```python
from build123d import *

# Parameters (mm, degrees)
SKETCH1_W           = 86.36
SKETCH1_H           = 76.2
SKETCH1_R           = 2.2225
SKETCH1_W_2         = 8.255
SKETCH1_R_2         = 1.016
BOSS_EXTRUDE1_DEPTH = 3.175
SKETCH2_W           = 102.87
SKETCH2_H           = 76.2
SKETCH2_W_2         = 100.33
SKETCH2_H_2         = 72.39
BOSS_EXTRUDE3_DEPTH = 12.7


with BuildPart() as part:
    # Sketch1 → Boss-Extrude1 (new body)
    # profile 1 of 3: a face of its own
    with BuildSketch(Plane(origin=(0, 0, 0), x_dir=(1, 0, 0), z_dir=(0, 1, 0))):
        Rectangle(SKETCH1_W, SKETCH1_H)
        with Locations(Location((-38.1, -10.16, 0), (0, 0, 270))):
            Circle(SKETCH1_R, mode=Mode.SUBTRACT)
        with Locations(Location((-38.1, 10.16, 0), (0, 0, 270))):
            Circle(SKETCH1_R, mode=Mode.SUBTRACT)
        with Locations(Location((38.1, -10.16, 0), (0, 0, 270))):
            Circle(SKETCH1_R, mode=Mode.SUBTRACT)
        with Locations(Location((38.1, 10.16, 0), (0, 0, 270))):
            Circle(SKETCH1_R, mode=Mode.SUBTRACT)
    # profile 2 of 3: a face of its own
    with BuildSketch(Plane(origin=(0, 0, 0), x_dir=(1, 0, 0), z_dir=(0, 1, 0))):
        with Locations((-47.3075, 0)):
            Rectangle(SKETCH1_W_2, SKETCH1_H)
        with Locations(Location((-46.355, 31.369, 0), (0, 0, 270))):
            Circle(SKETCH1_R_2, mode=Mode.SUBTRACT)
        with Locations(Location((-46.355, -31.369, 0), (0, 0, 270))):
            Circle(SKETCH1_R_2, mode=Mode.SUBTRACT)
    # profile 3 of 3: a face of its own
    with BuildSketch(Plane(origin=(0, 0, 0), x_dir=(1, 0, 0), z_dir=(0, 1, 0))):
        with Locations((47.3075, 0)):
            Rectangle(SKETCH1_W_2, SKETCH1_H)
        with Locations(Location((46.355, -31.369, 0), (0, 0, 270))):
            Circle(SKETCH1_R_2, mode=Mode.SUBTRACT)
        with Locations(Location((46.355, 31.369, 0), (0, 0, 270))):
            Circle(SKETCH1_R_2, mode=Mode.SUBTRACT)
    extrude(amount=BOSS_EXTRUDE1_DEPTH)

    # Sketch2 → Boss-Extrude3 (add)
    with BuildSketch(Plane(origin=(0, 3.175, 0), x_dir=(1, 0, 0), z_dir=(0, 1, 0))):
        Rectangle(SKETCH2_W, SKETCH2_H)
        Rectangle(SKETCH2_W_2, SKETCH2_H_2, mode=Mode.SUBTRACT)
    extrude(amount=BOSS_EXTRUDE3_DEPTH)


solid = part.part
```
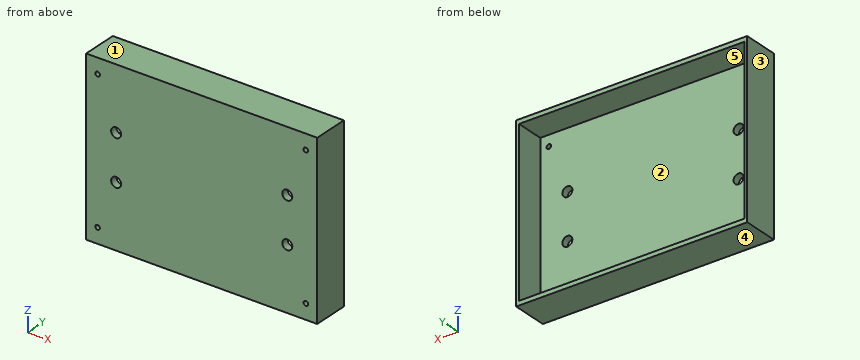
For this review, take the finished solid that the model builds, in its own axes (mm). Face numbers are marked on the shaded views. A direction names the side the tool comes from. Round coordinates to 2 decimals unless told otherwise and drop trailing zeros. Write each loop counter-clockwise with the first axis right and the second up, starting at its lowest first coordinate (ties: lowest second). Pieces come first, ordered by that corner, then holes. Notation, with made-up numbers: (-35, 12.25) - (-14, 12.25) arc R6 cw to (-14, 18.25) - close; hole circle Ø5 at (6, 35). An arc over 180 degrees is marked (long way). Put each result on its own line as item: value.
Q1. Machinability: for the marked faces 4 and 5, which of the approach directions +Z, -Z, +X, -X, +Y, -Y give a long, thin tool a straight path to every point of the face, cutting with its end or side? Answer none if there is none.
Solved:
face 4: -Z, +X, -X, +Y, -Y
face 5: +Y
Q2. We need section A-A (x = -38.1). Give the boundary of the cut face in (y, z) (1 decimal), and give its area (3 significant figures).
Solved:
outline: (0, -38.1) - (15.9, -38.1) - (15.9, -36.2) - (3.2, -36.2) - (3.2, -12.4) - (0, -12.4) - close; (0, -7.9) - (3.2, -7.9) - (3.2, 7.9) - (0, 7.9) - close; (0, 12.4) - (3.2, 12.4) - (3.2, 36.2) - (15.9, 36.2) - (15.9, 38.1) - (0, 38.1) - close
area: 262 mm2
Q3. Insertion check: pin 1 Ø6 at (x, z) = (38.1, 10.16) entering from +Y (3 decimals). The pin has a flat end and moves straight along its axis. Give the tip position at first contact, or say it passes through.
Solved:
pin 1: stops at y = 3.175
Q4. Wall thickness on probe 1 along X at (y, z) = (1.1, 10.16) (1 decimal); probe 2 along Z at (x, y) = (41.5, 11) (3 decimals); probe 3 along X at (y, z) = (4.25, -6) (3 decimals): over which ranges is each line inside the solid? List them lowest first.
Solved:
probe 1: x = -51.4 to -40.3, -35.9 to 35.9, 40.3 to 51.4
probe 2: z = -38.1 to -36.195, 36.195 to 38.1
probe 3: x = -51.435 to -50.165, 50.165 to 51.435
Q5. We need section D-D (x = 0). Give the boundary of the cut face in (y, z) (3 decimals).
Solved:
outline: (0, -38.1) - (15.875, -38.1) - (15.875, -36.195) - (3.175, -36.195) - (3.175, 36.195) - (15.875, 36.195) - (15.875, 38.1) - (0, 38.1) - close
Q6. We need section B-B (z = -10.16). Give the boundary of the cut face in (x, y) (1 decimal), and give its area (3 significant figures).
Solved:
outline: (-51.4, 0) - (-40.3, 0) - (-40.3, 3.2) - (-50.2, 3.2) - (-50.2, 15.9) - (-51.4, 15.9) - close; (-35.9, 0) - (35.9, 0) - (35.9, 3.2) - (-35.9, 3.2) - close; (40.3, 0) - (51.4, 0) - (51.4, 15.9) - (50.2, 15.9) - (50.2, 3.2) - (40.3, 3.2) - close
area: 331 mm2
Q7. We need section C-C (y = 9). Give the boundary of the cut face in (x, z) (3 decimals).
Solved:
outline: (-51.435, -38.1) - (51.435, -38.1) - (51.435, 38.1) - (-51.435, 38.1) - close; hole (-50.165, -36.195) - (50.165, -36.195) - (50.165, 36.195) - (-50.165, 36.195) - close
Q8. Mouldability with a two-part tool opening along X and no side actions: class the marked faces 1, 2 and 3 as released by +X, released by -X, zero draft, split by the parting line, or undercut.
Solved:
face 1: zero draft
face 2: undercut
face 3: released by -X
